```python
from build123d import *

# Parameters (mm, degrees)
SKETCH2_W           = 30
SKETCH2_H           = 30
BOSS_EXTRUDE1_DEPTH = 50
SKETCH3_W           = 25
SKETCH3_H           = 25
CUT_EXTRUDE1_DEPTH  = 2.5
FILLET1_R           = 5
SKETCH9_R           = 19.95304153
CUT_EXTRUDE2_DEPTH  = 5


with BuildPart() as part:
    # Sketch2 → Boss-Extrude1 (new body)
    with BuildSketch(Plane(origin=(0, 0, 0), x_dir=(1, 0, 0), z_dir=(0, 1, 0))):
        Rectangle(SKETCH2_W, SKETCH2_H)
    extrude(amount=BOSS_EXTRUDE1_DEPTH)

    # Sketch3 → Cut-Extrude1 (cut)
    with BuildSketch(Plane(origin=(0, 50, 0), x_dir=(1, 0, 0), z_dir=(0, 1, 0))):
        Rectangle(SKETCH3_W, SKETCH3_H)
    extrude(amount=-CUT_EXTRUDE1_DEPTH, mode=Mode.SUBTRACT)

    # Fillet1
    fillet1_edges = [part.edges().sort_by_distance(p)[0] for p in [
        (15, 25, 15),
        (-15, 25, 15),
        (-15, 25, -15),
        (15, 25, -15),
    ]]
    fillet(fillet1_edges, radius=FILLET1_R)

    # Cut-Loft2: read off the stored shape, not the designer's step
    # Cut-Loft2: loft between two sections, ruled curve by curve
    cut_loft2_from = [
        Edge.make_bspline([(0, 0, -12.5), (-25, 0, -12.5), (-25, 0, 12.5), (0, 0, 12.5), (25, 0, 12.5), (25, 0, -12.5), (0, 0, -12.5)], [0, 0, 0, 0, 0.5, 0.5, 0.5, 1, 1, 1, 1], 3, [1, 0.333333333, 0.333333333, 1, 0.333333333, 0.333333333, 1]),
    ]
    cut_loft2_to = [
        Edge.make_bspline([(0.784484005, 47.5, -2.373728048), (-3.962972092, 47.5, -3.942696057), (-5.531940101, 47.5, 0.804760039), (-0.784484005, 47.5, 2.373728048), (3.962972092, 47.5, 3.942696057), (5.531940101, 47.5, -0.804760039), (0.784484005, 47.5, -2.373728048)], [0, 0, 0, 0, 0.5, 0.5, 0.5, 1, 1, 1, 1], 3, [1, 0.333333333, 0.333333333, 1, 0.333333333, 0.333333333, 1]),
    ]
    cut_loft2 = Solid(Shell([*[Face.make_surface_from_curves(cut_loft2_from[k], cut_loft2_to[k]) for k in range(1)], Face(Wire(cut_loft2_from)), Face(Wire(cut_loft2_to))]))
    add(cut_loft2, mode=Mode.SUBTRACT)

    # Sketch9 → Cut-Extrude2 (cut)
    with BuildSketch(Plane(origin=(0, 35, 0), x_dir=(1, 0, 0), z_dir=(0, 1, 0))):
        Circle(SKETCH9_R)
        with BuildLine():
            Line((12.5, -10), (12.5, 10))
            ThreePointArc((12.5, 10), (11.767766953, 11.767766953), (10, 12.5))
            Line((10, 12.5), (-10, 12.5))
            ThreePointArc((-10, 12.5), (-11.767766953, 11.767766953), (-12.5, 10))
            Line((-12.5, 10), (-12.5, -10))
            ThreePointArc((-12.5, -10), (-11.767766953, -11.767766953), (-10, -12.5))
            Line((-10, -12.5), (10, -12.5))
            ThreePointArc((10, -12.5), (11.767766953, -11.767766953), (12.5, -10))
        make_face(mode=Mode.SUBTRACT)
    extrude(amount=CUT_EXTRUDE2_DEPTH, mode=Mode.SUBTRACT)


solid = part.part
```
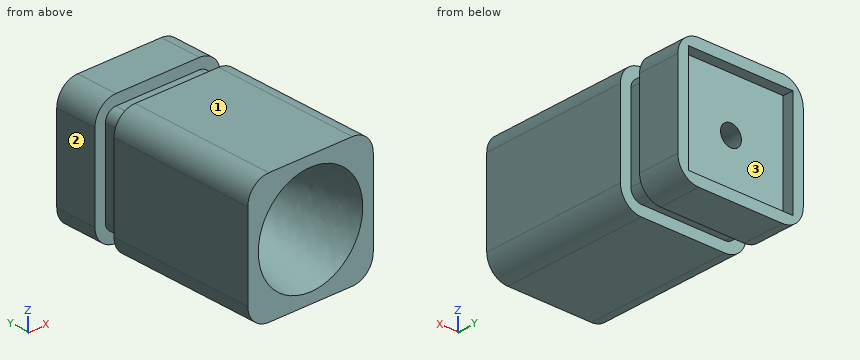
CAD build for the part. Positions are in the model's coordinates, mm. Face numbers are marked on the shaded views. Coordinates: 2 decimals unless noted, no trailing zeros.
(1) Pin check, flat tips, straight feed: pin 1 Ø6 at (x, z) = (6.5, 1) entering from +Y; pin 2 Ø1.5 at (y, z) = (38.5, -4) entering from +X; pin 3 Ø1.5 at (x, y) = (4.5, 37.5) entering from +Z. Stop position of each tip, or through.
Solution:
pin 1: stops at y = 47.5
pin 2: stops at x = 12.5
pin 3: stops at z = 12.5
(2) Mould opens along Z. For the marked faces 1, 2 and 3 say: released by +Z, released by -Z, zero draft, split by the parting line, or undercut.
Solution:
face 1: released by +Z
face 2: zero draft
face 3: undercut
(3) Drill centre lines: L1, parallel to Y at x = 5, z = 14; L2, parallel to Y at x = 11.5, z = -7; L3, parallel to X at y = 38, z = 8.5. Where is each one in solid material? Low to high.
Solution:
L1: y = 0 to 35, 40 to 50
L2: y = 0 to 47.5
L3: x = -12.5 to 12.5
